Autodesk Inventor part; units mm, degrees
ref_plane "YZ Plane" through (0, 0, 0) normal (1, 0, 0) x (0, 1, 0)
ref_plane "XZ Plane" through (0, 0, 0) normal (0, 1, 0) x (-1, 0, 0)
ref_plane "XY Plane" through (0, 0, 0) normal (0, 0, 1) x (1, 0, 0)
sketch "Sketch1" plane through (0, 0, 0) normal (0, 0, 1) x (1, 0, 0)
  line L0 (0, 0) -> (-15, 0)
  line L1 (-15, 0) -> (-15, 5.9)
  line L2 (-15, 5.9) -> (0, 5.9)
  line L3 (0, 5.9) -> (0, 0)
  dimension "d0" = 5.9
  dimension "d1" = 15
extrude "Extrusion1" add sketch "Sketch1" along normal blind 4
sketch "Sketch2" plane through (-15, 5.9, 0) normal (0, 1, 0) x (1, 0, 0)
  circle A0 centre (12.5, -2) radius 1.025
  circle A1 centre (2.5, -2) radius 1.025
  line L0 (15, 0) -> (15, -4)
  line L1 (15, -4) -> (0, -4)
  dimension "d4" = 10
  dimension "d5" = 2.5
  dimension "d6" = 2
  dimension "d7" = 2
  dimension "d8" = 2.05
  dimension "d9" = 2.05
extrude "Extrusion2" cut sketch "Sketch2" against normal blind 8
sketch "Sketch3" plane through (0, 0, 0) normal (0, 0, -1) x (-1, 0, 0)
  line L0 (0, 0) -> (0, 5.9)
  line L1 (0, 0) -> (-10, 0)
  line L2 (-10, 0) -> (-10, 5.9)
  line L3 (-10, 5.9) -> (0, 5.9)
  line L4 (0, 5.9) -> (0, 0)
  dimension "d12" = 10
extrude "Extrusion3" add sketch "Sketch3" against normal blind 4
sketch "Sketch4" plane through (0, 0, 0) normal (0, 0, -1) x (-1, 0, 0)
  line L0 (3.525, 5.9) -> (3.525, 0)
  line L1 (1.475, 5.9) -> (1.475, 0)
  circle A0 centre (-3, 1.9) radius 1.025
  circle A1 centre (-8, 1.9) radius 1.025
  line L2 (-10, 5.9) -> (15, 5.9)
  line L3 (15, 0) -> (-10, 0)
  line L4 (-10, 5.9) -> (-10, 0)
  point P0 (0, 0)
  dimension "d15" = 2.05
  dimension "d16" = 5.9
  dimension "d17" = 4
  dimension "d18" = 4
  dimension "d19" = 5
  dimension "d20" = 2
  dimension "d21" = 2.05
  dimension "d22" = 2.05
extrude "Extrusion4" cut sketch "Sketch4" against normal blind 4 contours A0 | A1
equation "\"d7\" = d6"
equation "\"d18\" = d17"
equation "\"d21\" = d15"
equation "\"d22\" = d15"
properties part number "AngleScrewBlocActuator" material "Stainless Steel"
Geometry: final body of the model. Coordinates: model frame, mm. Coordinates: 2 decimals unless noted, no trailing zeros. Loops run counter-clockwise (first coordinate to the right, second up) from the corner with the lowest first, then second, coordinate; pieces in that order, holes last. Notation, with made-up numbers: (53, -10.5) -> (93, -10.5) arc R19 ccw to (93, 13.5) -> close; hole circle Ø6 at (39.5, -5). An arc over 180 degrees is marked (long way). Use a Markdown table: item, result. Add a question column.
(1) Section query B-B, the plane y = 1.6. Return loops of the section in (x, z) (3 decimals), plus the area to 3 significant figures.
(2) Line query: line 1 along Z through (x, y) = (-12.5, 2) (3 decimals); line 2 along X through (y, z) = (4, 2) (3 decimals); line 3 along X through (y, z) = (1.8, 1.95). Output: solid intervals per line, ascending.
(3) Section query A-A, the plane z = 2. Return loops of the section in (x, y) (3 decimals), plus the area to 3 significant figures.
(4) Section query C-C, the plane x = 8. Return loops of the section in (y, z) (3 decimals).
(5) Mould query, pull axis X, two halves, no side actions, for faces 1 (the flat face through (10, 3, 2)), 2 (the cylindrical face through (3.813, 1.276, 1.972)), 3 (the flat face through (-2.7, 0, 3.3)). Classes: pulls with the +X half, pulls with the -X half, needs draft (parallel to the pull), parting line crosses it, or undercut.
(6) Section query D-D, the plane y = 0.4. Return loops of the section in (x, z) (3 decimals), plus the area to 3 significant figures.
Answer:
| question | item | result |
|---|---|---|
| 1 | outline | (-15, 0) -> (2.02, 0) -> (2.02, 4) -> (-15, 4) -> close; (3.98, 0) -> (7.02, 0) -> (7.02, 4) -> (3.98, 4) -> close; (8.98, 0) -> (10, 0) -> (10, 4) -> (8.98, 4) -> close; hole circle Ø2.05 at (-12.5, 2); hole circle Ø2.05 at (-2.5, 2) |
| 1 | area | 77.7 mm^2 |
| 2 | line 1 | z = 0 to 0.975, 3.025 to 4 |
| 2 | line 2 | x = -15 to -13.525, -11.475 to -3.525, -1.475 to 10 |
| 2 | line 3 | x = -15 to -13.52, -11.48 to -3.52, -1.48 to 1.98, 4.02 to 6.98, 9.02 to 10 |
| 3 | outline | (-15, 0) -> (-13.525, 0) -> (-13.525, 5.9) -> (-15, 5.9) -> close; (-11.475, 0) -> (-3.525, 0) -> (-3.525, 5.9) -> (-11.475, 5.9) -> close; (-1.475, 0) -> (10, 0) -> (10, 5.9) -> (-1.475, 5.9) -> close; hole circle Ø2.05 at (3, 1.9); hole circle Ø2.05 at (8, 1.9) |
| 3 | area | 117 mm^2 |
| 4 | outline | (0, 0) -> (0.875, 0) -> (0.875, 4) -> (0, 4) -> close; (2.925, 0) -> (5.9, 0) -> (5.9, 4) -> (2.925, 4) -> close |
| 5 | face 1 | pulls with the +X half |
| 5 | face 2 | undercut |
| 5 | face 3 | needs draft |
| 6 | outline | (-15, 0) -> (10, 0) -> (10, 4) -> (-15, 4) -> close; hole circle Ø2.05 at (-12.5, 2); hole circle Ø2.05 at (-2.5, 2) |
| 6 | area | 93.4 mm^2 |
